Work out the finished part from the listing and answer in its coordinate system (mm). A direction names the side the tool comes from. Coordinates: 2 decimals unless noted, no trailing zeros. Write each loop counter-clockwise with the first axis right and the second up, starting at its lowest first coordinate (ties: lowest second). Pieces come first, ordered by that corner, then holes. Notation, with made-up numbers: (15.25, 56.25) - (69.25, 56.25) arc R10 cw to (69.25, 63.25) - close; hole circle Ø10 at (-32.75, -39). An arc over 180 degrees is marked (long way). Answer as a JSON object with one key per item and string values. Group by question number.
from build123d import *

# Parameters (mm, degrees)
SKETCH1_W               = 50
SKETCH1_H               = 80
BOSS_EXTRUDE1_DEPTH     = 10
SKETCH2_R               = 2.25
CUT_EXTRUDE1_DEPTH      = 49.218253805
CHAMFER1_SIZE           = 2
BOSS_EXTRUDE2_DEPTH     = 40
CUT_EXTRUDE2_DEPTH      = 68.19064295
CUT_EXTRUDE2_DEPTH_BACK = 68.19064295
SKETCH4_W               = 28
SKETCH4_H               = 5
CUT_EXTRUDE3_REACH      = 92.091
SKETCH5_W               = 13
SKETCH5_H               = 8
FILLET1_R               = 1
FILLET2_R               = 2


with BuildPart() as part:
    # Sketch1 → Boss-Extrude1 (new body)
    with BuildSketch(Plane(origin=(0, 0, 0), x_dir=(1, 0, 0), z_dir=(0, 1, 0))):
        Rectangle(SKETCH1_W, SKETCH1_H)
    extrude(amount=BOSS_EXTRUDE1_DEPTH)

    # Sketch2 → Cut-Extrude1 (cut, through all)
    with BuildSketch(Plane(origin=(0, 10, 0), x_dir=(1, 0, 0), z_dir=(0, 1, 0))):
        with Locations(Location((-14.730430452, 0, 0), (0, 0, 270))):
            Circle(SKETCH2_R)
        with Locations(Location((-14.730430452, 25, 0), (0, 0, 270))):
            Circle(SKETCH2_R)
        with Locations(Location((-14.730430452, -25, 0), (0, 0, 270))):
            Circle(SKETCH2_R)
        with Locations(Location((14.730430452, -25, 0), (0, 0, 90))):
            Circle(SKETCH2_R)
        with Locations(Location((14.730430452, 0, 0), (0, 0, 90))):
            Circle(SKETCH2_R)
        with Locations(Location((14.730430452, 25, 0), (0, 0, 90))):
            Circle(SKETCH2_R)
    extrude(amount=-CUT_EXTRUDE1_DEPTH, mode=Mode.SUBTRACT)

    # Chamfer1
    chamfer1_edges = [part.edges().sort_by_distance(p)[0] for p in [
        (-14.730430452, 10, -27.25),
        (-14.730430452, 10, 22.75),
        (14.730430452, 10, 27.25),
        (14.730430452, 10, 2.25),
        (14.730430452, 10, -22.75),
        (-14.730430452, 10, -2.25),
    ]]
    chamfer(chamfer1_edges, length=CHAMFER1_SIZE)

    # Sketch3 → Boss-Extrude2 (add, symmetric)
    with BuildSketch(Plane.XY):
        Polygon((-25, 10), (-32.65, 10), (-32.65, 39.4), (-24.65, 39.4), (-24.65, 41.4), (-34.65, 41.4), (-34.65, 8), (-25, 0), align=None)
        Polygon((34.65, 8), (25, 0), (25, 10), (32.65, 10), (32.65, 39.4), (24.65, 39.4), (24.65, 41.4), (34.65, 41.4), align=None)
    extrude(amount=BOSS_EXTRUDE2_DEPTH, both=True)

    # Sketch4 → Cut-Extrude2 (cut, two sides: drawn at the far end of the back side and taken through both)
    with BuildSketch(Plane(origin=(0, 0, 0), x_dir=(0, 0, -1), z_dir=(1, 0, 0)).offset(-CUT_EXTRUDE2_DEPTH_BACK)):
        with Locations((-26, 38.9)):
            Rectangle(SKETCH4_W, SKETCH4_H)
    extrude(amount=CUT_EXTRUDE2_DEPTH + CUT_EXTRUDE2_DEPTH_BACK, mode=Mode.SUBTRACT)

    # Sketch5 → Cut-Extrude3 (cut, up to next)
    with BuildSketch(Plane(origin=(34.65, 0, 0), x_dir=(0, 0, -1), z_dir=(1, 0, 0)), mode=Mode.PRIVATE) as cut_extrude3_sk1:
        with Locations((31.5, 27)):
            Rectangle(SKETCH5_W, SKETCH5_H)
    cut_extrude3_tool1 = extrude(cut_extrude3_sk1.sketch, amount=-CUT_EXTRUDE3_REACH, mode=Mode.PRIVATE) & part.part
    add(cut_extrude3_tool1.solids().sort_by_distance((34.65, 27, -31.5))[0], mode=Mode.SUBTRACT)

    # Fillet1
    fillet1_edges = [part.edges().sort_by_distance(p)[0] for p in [
        (32.65, 23.2, 40),
        (32.65, 37.9, 12),
        (24.65, 39.4, -14),
        (-24.65, 39.4, -14),
        (-28.65, 39.4, 12),
        (-32.65, 37.9, 12),
        (28.65, 39.4, 12),
        (0, 10, 40),
        (-32.65, 24.7, -40),
        (-28.65, 39.4, -40),
        (-32.65, 23.2, 40),
        (0, 10, -40),
        (28.65, 39.4, -40),
        (32.65, 24.7, -40),
    ]]
    fillet(fillet1_edges, radius=FILLET1_R)

    # Fillet2
    # the kernel refuses this fillet: 2 mm, written as the material it takes off along each edge
    with BuildSketch(Plane(origin=(-24.278787146, 2, 38), x_dir=(0, -1, 0), z_dir=(0, 0, 1))) as fillet2_piece_1_section:
        Polygon((0, 0), (FILLET2_R * 1.02, 0), (FILLET2_R * 1.02, -FILLET2_R * 0.367818555432), (FILLET2_R * 0.785250632337, -FILLET2_R * 0.650984980176), align=None)
    fillet2_piece_1 = extrude(amount=FILLET2_R * 1.02, mode=Mode.PRIVATE)
    fillet2_piece_1 = fillet2_piece_1 - Plane(origin=(-24.278787146, 2, 38), x_dir=(0.3392244381566016, 0.9407054696116836, 0), z_dir=(0, 0, 1)) * Sphere(FILLET2_R, mode=Mode.PRIVATE)
    add(fillet2_piece_1, mode=Mode.SUBTRACT)
    with BuildSketch(Plane(origin=(24.278787146, 2, -38), x_dir=(0, -1, 0), z_dir=(0, 0, -1))) as fillet2_piece_2_section:
        Polygon((0, 0), (FILLET2_R * 1.02, 0), (FILLET2_R * 1.02, -FILLET2_R * 0.367818555432), (FILLET2_R * 0.785250632337, -FILLET2_R * 0.650984980176), align=None)
    fillet2_piece_2 = extrude(amount=FILLET2_R * 1.02, mode=Mode.PRIVATE)
    fillet2_piece_2 = fillet2_piece_2 - Plane(origin=(24.278787146, 2, -38), x_dir=(-0.3392244381566016, 0.9407054696116836, 0), z_dir=(0, 0, -1)) * Sphere(FILLET2_R, mode=Mode.PRIVATE)
    add(fillet2_piece_2, mode=Mode.SUBTRACT)
    with BuildSketch(Plane(origin=(24.278787146, 2, 38), x_dir=(0, -1, 0), z_dir=(0, 0, 1))) as fillet2_piece_3_section:
        Polygon((0, 0), (FILLET2_R * 1.02, 0), (FILLET2_R * 1.02, FILLET2_R * 0.367818555432), (FILLET2_R * 0.785250632337, FILLET2_R * 0.650984980176), align=None)
    fillet2_piece_3 = extrude(amount=FILLET2_R * 1.02, mode=Mode.PRIVATE)
    fillet2_piece_3 = fillet2_piece_3 - Plane(origin=(24.278787146, 2, 38), x_dir=(-0.3392244381566016, 0.9407054696116836, 0), z_dir=(0, 0, 1)) * Sphere(FILLET2_R, mode=Mode.PRIVATE)
    add(fillet2_piece_3, mode=Mode.SUBTRACT)
    with BuildSketch(Plane(origin=(-24.278787146, 2, -38), x_dir=(0, -1, 0), z_dir=(0, 0, -1))) as fillet2_piece_4_section:
        Polygon((0, 0), (FILLET2_R * 1.02, 0), (FILLET2_R * 1.02, FILLET2_R * 0.367818555432), (FILLET2_R * 0.785250632337, FILLET2_R * 0.650984980176), align=None)
    fillet2_piece_4 = extrude(amount=FILLET2_R * 1.02, mode=Mode.PRIVATE)
    fillet2_piece_4 = fillet2_piece_4 - Plane(origin=(-24.278787146, 2, -38), x_dir=(0.3392244381566016, 0.9407054696116836, 0), z_dir=(0, 0, -1)) * Sphere(FILLET2_R, mode=Mode.PRIVATE)
    add(fillet2_piece_4, mode=Mode.SUBTRACT)
    with BuildSketch(Plane(origin=(-38.499267806, 11.191102844, 40), x_dir=(0.6382205687997308, 0.7698535611146761, -3.5527136788005e-15), z_dir=(0.7698535611146761, -0.6382205687997308, 0)), Plane(origin=(-38.499267806, 11.191102844, -40), x_dir=(0, 0, 1), z_dir=(0.7698535611146761, -0.6382205687997308, 0))) as fillet2_piece_5:
        with BuildLine():
            CenterArc((FILLET2_R, -FILLET2_R), FILLET2_R, 90, 90)
            Line((0, -FILLET2_R), (-FILLET2_R * 0.02, -FILLET2_R))
            Line((-FILLET2_R * 0.02, -FILLET2_R), (-FILLET2_R * 0.02, FILLET2_R * 0.02))
            Line((-FILLET2_R * 0.02, FILLET2_R * 0.02), (FILLET2_R, FILLET2_R * 0.02))
            Line((FILLET2_R, FILLET2_R * 0.02), (FILLET2_R, 0))
        make_face()
    extrude(amount=16.813638561, mode=Mode.SUBTRACT)
    with BuildSketch(Plane(origin=(38.499267806, 11.191102844, -40), x_dir=(0, 0, 1), z_dir=(-0.7698535611146761, -0.6382205687997308, 0)), Plane(origin=(38.499267806, 11.191102844, 40), x_dir=(-0.6382205687997308, 0.7698535611146761, -3.5527136788005e-15), z_dir=(-0.7698535611146761, -0.6382205687997308, 0))) as fillet2_piece_6:
        with BuildLine():
            CenterArc((FILLET2_R, FILLET2_R), FILLET2_R, 180, 90)
            Line((0, FILLET2_R), (-FILLET2_R * 0.02, FILLET2_R))
            Line((-FILLET2_R * 0.02, FILLET2_R), (-FILLET2_R * 0.02, -FILLET2_R * 0.02))
            Line((-FILLET2_R * 0.02, -FILLET2_R * 0.02), (FILLET2_R, -FILLET2_R * 0.02))
            Line((FILLET2_R, -FILLET2_R * 0.02), (FILLET2_R, 0))
        make_face()
    extrude(amount=16.813638561, mode=Mode.SUBTRACT)
    with BuildSketch(Plane(origin=(-24.278787146, 0, -40), x_dir=(0, 0, 1), z_dir=(1, 0, 0)), Plane(origin=(24.278787146, 0, 40), x_dir=(0, 0, -1), z_dir=(-1, 0, 0))) as fillet2_piece_7:
        with BuildLine():
            CenterArc((FILLET2_R, -FILLET2_R), FILLET2_R, 90, 90)
            Line((0, -FILLET2_R), (-FILLET2_R * 0.02, -FILLET2_R))
            Line((-FILLET2_R * 0.02, -FILLET2_R), (-FILLET2_R * 0.02, FILLET2_R * 0.02))
            Line((-FILLET2_R * 0.02, FILLET2_R * 0.02), (FILLET2_R, FILLET2_R * 0.02))
            Line((FILLET2_R, FILLET2_R * 0.02), (FILLET2_R, 0))
        make_face()
    extrude(amount=48.557574292, mode=Mode.SUBTRACT)
    with BuildSketch(Plane(origin=(-34.65, 8, 42.349663946), x_dir=(0, 1, 0), z_dir=(0, 0, -1)), Plane(origin=(34.65, 8, -42.349663946), x_dir=(0, 1, 0), z_dir=(0, 0, 1))) as fillet2_piece_8:
        with BuildLine():
            CenterArc((FILLET2_R * 0.469932789135, FILLET2_R), FILLET2_R, 219.659259409, 50.340740591)
            Line((-FILLET2_R * 0.299920771979, FILLET2_R * 0.3617794312), (-FILLET2_R * 0.315317843202, FILLET2_R * 0.349015019824))
            Line((-FILLET2_R * 0.315317843202, FILLET2_R * 0.349015019824), (-FILLET2_R * 0.0093986557827, -FILLET2_R * 0.02))
            Line((-FILLET2_R * 0.0093986557827, -FILLET2_R * 0.02), (FILLET2_R * 0.469932789135, -FILLET2_R * 0.02))
            Line((FILLET2_R * 0.469932789135, -FILLET2_R * 0.02), (FILLET2_R * 0.469932789135, 0))
        make_face()
    extrude(amount=84.699327891, mode=Mode.SUBTRACT)
    with BuildSketch(Plane(origin=(25, 0, -38), x_dir=(-1, 0, 0), z_dir=(0, 0, 1)), Plane(origin=(-25, 0, 38), x_dir=(1, 0, 0), z_dir=(0, 0, -1))) as fillet2_piece_9:
        with BuildLine():
            CenterArc((FILLET2_R * 0.360606426894, -FILLET2_R), FILLET2_R, 90, 39.659259409)
            Line((-FILLET2_R * 0.277614141905, -FILLET2_R * 0.230146438885), (-FILLET2_R * 0.290378553281, -FILLET2_R * 0.214749367663))
            Line((-FILLET2_R * 0.290378553281, -FILLET2_R * 0.214749367663), (-FILLET2_R * 0.00721212853789, FILLET2_R * 0.02))
            Line((-FILLET2_R * 0.00721212853789, FILLET2_R * 0.02), (FILLET2_R * 0.360606426894, FILLET2_R * 0.02))
            Line((FILLET2_R * 0.360606426894, FILLET2_R * 0.02), (FILLET2_R * 0.360606426894, 0))
        make_face()
    extrude(amount=76, mode=Mode.SUBTRACT)


solid = part.part
Q1. Section D-D on z = -17 is taken. Determine the outline of the cut face in (x, y), plus the area to 3 significant figures.
Q2. Consider L1, parallel to X at y = 32.5, z = -25; L2, parallel to Z at x = 14, y = 9; L3, parallel to X at y = 6, z = 0. Determine where each line is inside the solid, lowest interval first. Write a range as from..to.
Q3. For a pull along Y with two mould halves and no side action, classify faces 4 (the face through (29.8, 3.98, 0.53)), 5 (the face through (29, 39.4, -14)), 6 (the face through (-31, 41, 12)) as +Y half, -Y half, draft (parallel to the pull), parting line (faces both ways), or undercut.
Q4. A tool of negligible diameter and unlimited length cuts with its end or side. For faces 1 (the face through (30, 41.4, -14)), 2 (the face through (0, 10, 1)), 3 (the face through (34, 27, -25)), from which of +Z, -Z, +X, -X, +Y, -Y can it reach the whole face along a straight path? Write none if from no direction.
Q5. Section B-B on y = 27 is taken. Determine the outline of the cut face in (x, z).
Q6. Section C-C on y = 17.5 is taken. Determine the outline of the cut face in (x, z).
Q7. Flat-ended cylindrical pins translate along their axes: pin 1 Ø1 at (x, z) = (34, -34) entering from -Y; pin 2 Ø2 at (x, z) = (-26.5, -32) entering from -Y; pin 3 Ø1 at (x, z) = (34, 21) entering from +Y. Find the tip coordinate at first contact, or state that the pin passes through.
Q8. Section A-A on z = 25 is taken. Determine the outline of the cut face in (x, y), plus the area to 3 significant figures.
Numbers:
{
 "1": {"outline": "(-34.65, 8.94) arc R2 ccw to (-33.93, 7.4) - (-25.56, 0.46) arc R2 ccw to (-24.28, 0) - (24.28, 0) arc R2 ccw to (25.56, 0.46) - (33.93, 7.4) arc R2 ccw to (34.65, 8.94) - (34.65, 41.4) - (24.65, 41.4) - (24.65, 40.4) arc R1 ccw to (25.65, 39.4) - (32.65, 39.4) - (32.65, 10) - (-32.65, 10) - (-32.65, 39.4) - (-25.65, 39.4) arc R1 ccw to (-24.65, 40.4) - (-24.65, 41.4) - (-34.65, 41.4) - close", "area": "773 mm²"},
 "2": {"L1": "x = -34.65..-32.65, 32.65..34.65", "L2": "z = -40..-28.17, -21.83..-3.17, 3.17..21.83, 28.17..40", "L3": "x = -32.24..-16.98, -12.48..12.48, 16.98..32.24"},
 "3": {"face 4": "-Y half", "face 5": "undercut", "face 6": "draft"},
 "4": {"face 1": "+Z, -Z, +X, -X, +Y", "face 2": "+Z, -Z", "face 3": "+X"},
 "5": {"outline": "(-34.65, -40) - (-33.65, -40) arc R1 ccw to (-32.65, -39) - (-32.65, 39) arc R1 ccw to (-33.65, 40) - (-34.65, 40) - close; (32.65, -39) arc R1 ccw to (33.65, -40) - (34.65, -40) - (34.65, -38) - (32.65, -38) - close; (32.65, -25) - (34.65, -25) - (34.65, 40) - (33.65, 40) arc R1 ccw to (32.65, 39) - close"},
 "6": {"outline": "(-34.65, -40) - (-33.65, -40) arc R1 ccw to (-32.65, -39) - (-32.65, 39) arc R1 ccw to (-33.65, 40) - (-34.65, 40) - close; (32.65, -39) arc R1 ccw to (33.65, -40) - (34.65, -40) - (34.65, 40) - (33.65, 40) arc R1 ccw to (32.65, 39) - close"},
 "7": {"pin 1": "stops at y = 7.05", "pin 2": "stops at y = 0.42", "pin 3": "stops at y = 36.4"},
 "8": {"outline": "(-34.65, 8.94) arc R2 ccw to (-33.93, 7.4) - (-25.56, 0.46) arc R2 ccw to (-24.28, 0) - (-16.98, 0) - (-16.98, 8) - (-18.98, 10) - (-32.65, 10) - (-32.65, 36.4) - (-34.65, 36.4) - close; (-12.48, 0) - (12.48, 0) - (12.48, 8) - (10.48, 10) - (-10.48, 10) - (-12.48, 8) - close; (16.98, 0) - (24.28, 0) arc R2 ccw to (25.56, 0.46) - (33.93, 7.4) arc R2 ccw to (34.65, 8.94) - (34.65, 36.4) - (32.65, 36.4) - (32.65, 10) - (18.98, 10) - (16.98, 8) - close", "area": "623 mm²"}
}
